from build123d import *

# Parameters (mm, degrees)
SKETCH_1_W          = 60
SKETCH_1_H          = 90
EXTRUDE_1_DEPTH     = 3
SKETCH_2_R          = 1.65
CUT_EXTRUDE_1_DEPTH = 3
SKETCH_5_W          = 15.5
SKETCH_5_H          = 15.5
CUT_EXTRUDE_4_DEPTH = 1000
SKETCH_3_R          = 1.65
CUT_EXTRUDE_2_DEPTH = 3
SKETCH_4_R          = 6.75
CUT_EXTRUDE_3_DEPTH = 3
FILLET_1_R          = 2
SKETCH_6_W          = 69.11106811
SKETCH_6_H          = 12.862943276
CUT_EXTRUDE_5_DEPTH = 1000
FILLET_2_R          = 2
SKETCH_7_R          = 1.65
CUT_EXTRUDE_6_DEPTH = 1000


with BuildPart() as part:
    # 草图1 → 凸台-拉伸1 (new body)
    with BuildSketch(Plane.XY):
        Rectangle(SKETCH_1_W, SKETCH_1_H)
    extrude(amount=EXTRUDE_1_DEPTH)

    # 草图2 → 切除-拉伸1 (cut)
    with BuildSketch(Plane.XY.offset(3)):
        with Locations((0, 16)):
            Circle(SKETCH_2_R)
        with Locations((-8.227241336, 30.25)):
            Circle(SKETCH_2_R)
        with Locations((8.227241336, 30.25)):
            Circle(SKETCH_2_R)
    extrude(amount=-CUT_EXTRUDE_1_DEPTH, mode=Mode.SUBTRACT)

    # 草图5 → 切除-拉伸4 (cut)
    with BuildSketch(Plane.XY.offset(3)):
        with Locations((0, -10)):
            Rectangle(SKETCH_5_W, SKETCH_5_H)
    extrude(amount=-CUT_EXTRUDE_4_DEPTH, mode=Mode.SUBTRACT)

    # 草图3 → 切除-拉伸2 (cut)
    with BuildSketch(Plane.XY.offset(3)):
        with Locations((4.5, -27.75)):
            Circle(SKETCH_3_R)
        with Locations((-4.5, -27.75)):
            Circle(SKETCH_3_R)
    extrude(amount=-CUT_EXTRUDE_2_DEPTH, mode=Mode.SUBTRACT)

    # 草图4 → 切除-拉伸3 (cut)
    with BuildSketch(Plane.XY.offset(3)):
        with Locations((0, 25.5)):
            Circle(SKETCH_4_R)
    extrude(amount=-CUT_EXTRUDE_3_DEPTH, mode=Mode.SUBTRACT)

    # 圆角1
    fillet_1_edges = [part.edges().sort_by_distance(p)[0] for p in [
        (-30, 45, 1.5),
        (30, 45, 1.5),
    ]]
    fillet(fillet_1_edges, radius=FILLET_1_R)

    # 草图6 → 切除-拉伸5 (cut)
    with BuildSketch(Plane.XY.offset(3)):
        with Locations((0, -41.431471638)):
            Rectangle(SKETCH_6_W, SKETCH_6_H)
    extrude(amount=-CUT_EXTRUDE_5_DEPTH, mode=Mode.SUBTRACT)

    # 圆角2
    fillet_2_edges = [part.edges().sort_by_distance(p)[0] for p in [
        (30, -35, 1.5),
        (-30, -35, 1.5),
    ]]
    fillet(fillet_2_edges, radius=FILLET_2_R)

    # 草图7 → 切除-拉伸6 (cut)
    with BuildSketch(Plane.XY.offset(3)):
        with Locations((17.5, -5.5)):
            Circle(SKETCH_7_R)
        with Locations((17.5, -14.5)):
            Circle(SKETCH_7_R)
        with Locations((-17.5, -5.5)):
            Circle(SKETCH_7_R)
        with Locations((-17.5, -14.5)):
            Circle(SKETCH_7_R)
    extrude(amount=-CUT_EXTRUDE_6_DEPTH, mode=Mode.SUBTRACT)


solid = part.part
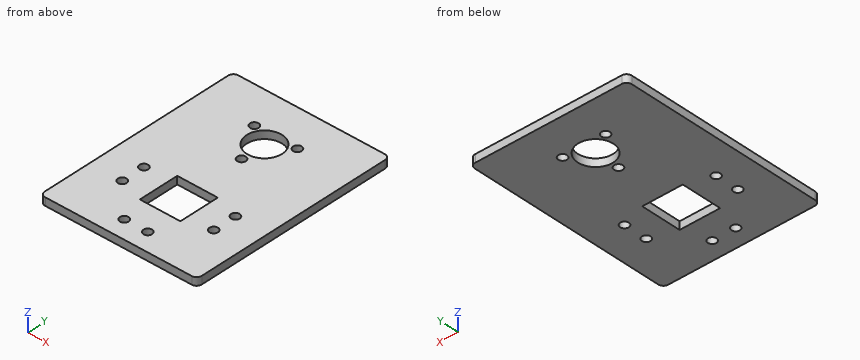
Geometry check sheet. Reference: the model listing, model coordinates, mm. Give positions to 0.01 mm unless a question says otherwise; leave off trailing zeros. Order: outer loops, then holes, each group sorted by start corner. A loop starts at its lowest first (then second) coordinate and runs counter-clockwise, first axis right, second up.
1) Cross-section at D-D (z = 0.55). Give the number of separate pieces and of enclosed holes in the cut face, then the cut area to 3 significant figures.
Results are:
separate pieces: 1
enclosed holes: 11
area: 4,340 mm2
2) Cross-section at B-B (x = 17.5). Record the boundary of the cut face in (y, z), then the cut area to 3 significant figures.
Results are:
outline: (-35, 0) - (-16.15, 0) - (-16.15, 3) - (-35, 3) - close; (-12.85, 0) - (-7.15, 0) - (-7.15, 3) - (-12.85, 3) - close; (-3.85, 0) - (45, 0) - (45, 3) - (-3.85, 3) - close
area: 220 mm2
3) Cross-section at C-C (y = -27.75). Record the boundary of the cut face in (x, z), then the cut area to 3 significant figures.
Results are:
outline: (-30, 0) - (-6.15, 0) - (-6.15, 3) - (-30, 3) - close; (-2.85, 0) - (2.85, 0) - (2.85, 3) - (-2.85, 3) - close; (6.15, 0) - (30, 0) - (30, 3) - (6.15, 3) - close
area: 160 mm2
4) Cross-section at A-A (y = 16). Record the boundary of the cut face in (x, z), then the cut area to 3 significant figures.
Results are:
outline: (-30, 0) - (-1.65, 0) - (-1.65, 3) - (-30, 3) - close; (1.65, 0) - (30, 0) - (30, 3) - (1.65, 3) - close
area: 170 mm2
5) Material ranges on probe 1 along Y at (x, z) = (17.5, 1.4); probe 2 along X at (y, z) = (-28, 0.5); probe 3 along X at (y, z) = (-3, 0.2), recorded low to high.
Results are:
probe 1: y = -35 to -16.15, -12.85 to -7.15, -3.85 to 45
probe 2: x = -30 to -6.13, -2.87 to 2.87, 6.13 to 30
probe 3: x = -30 to -7.75, 7.75 to 30
6) Gauge pin test, flat end, axial feed: pin 1 (2.5 mm diameter, centred on x = -4.5, y = -27.75, fed in from +Z). Record the tip position at first contact, or that the pin passes through.
Results are:
pin 1: passes through
